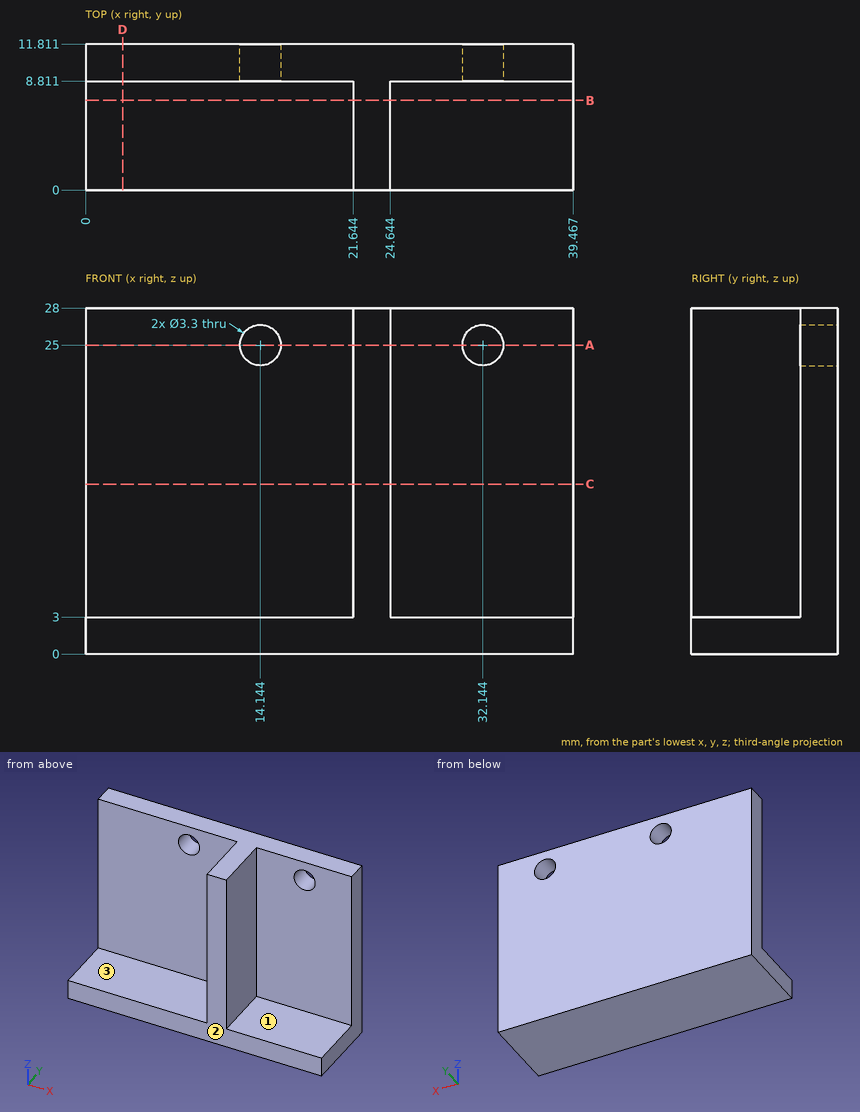
Study the drawing (mm; zero at the part's minimum x, y, z) and answer. A direction names the side the tool comes from. Coordinates: 2 decimals unless noted, no trailing zeros. Write each loop counter-clockwise with the first axis right and the second up, starting at its lowest first coordinate (ties: lowest second). Pieces come first, ordered by that corner, then holes. Notation, with made-up numbers: (-35.5, 67) - (-9.5, 67) arc R16 ccw to (-9.5, 82) - close; hole circle Ø6 at (59, 31). An arc over 180 degrees is marked (long way). Return JSON: item names as keys, results as strings. Group by question number.
1. Given pin 1 (4.5 mm diameter, centred on y = 5, z = 17, fed in from +X); pin 2 (2.5 mm diameter, centred on y = 2.5, z = 20.5, fed in from -X); pin 3 (5.5 mm diameter, centred on x = 32.14, z = 25, fed in from -Y); pin 4 (4.5 mm diameter, centred on x = 14.14, z = 25, fed in from +Y), each flat-ended and moving along its own axis, determine where each tip first touches the part or whether it passes through.
2. A cutting plane is placed at A-A, the plane z = 25. Determine the outline of the cut face in (x, y) (1 decimal).
3. A cutting plane is placed at C-C, the plane z = 13.75. Determine the outline of the cut face in (x, y) (1 decimal), plus the area to 3 significant figures.
4. Which of the six approach directions +Z, -Z, +X, -X, +Y, -Y give full straight-line access (tool end or side, diameter ignored) to the marked faces 1, 2 and 3?
5. Straight lines are drawn through the part: L1, parallel to X at y = 10.75, z = 25 (1 decimal); L2, parallel to Y at x = 17.5, z = 23; L3, parallel to X at y = 4, z = 20.5 (1 decimal). For each, find the intervals that lie inside material, in ascending order.
6. A cutting plane is placed at D-D, the plane x = 3. Determine the outline of the cut face in (y, z).
7. A cutting plane is placed at B-B, the plane y = 7.25. Determine the outline of the cut face in (x, z) (1 decimal).
Ans:
{
 "1": {"pin 1": "x = 24.64", "pin 2": "x = 21.64", "pin 3": "y = 8.81", "pin 4": "y = 11.81"},
 "2": {"outline": "(0, 8.8) - (12.5, 8.8) - (12.5, 11.8) - (0, 11.8) - close; (15.8, 8.8) - (21.6, 8.8) - (21.6, 0) - (24.6, 0) - (24.6, 8.8) - (30.5, 8.8) - (30.5, 11.8) - (15.8, 11.8) - close; (33.8, 8.8) - (39.5, 8.8) - (39.5, 11.8) - (33.8, 11.8) - close"},
 "3": {"outline": "(0, 8.8) - (21.6, 8.8) - (21.6, 0) - (24.6, 0) - (24.6, 8.8) - (39.5, 8.8) - (39.5, 11.8) - (0, 11.8) - close", "area": "145 mm²"},
 "4": {"face 1": "+Z, +X, -Y", "face 2": "+Z, -Z, +X, -X, -Y", "face 3": "+Z, -X, -Y"},
 "5": {"L1": "0 to 12.5, 15.8 to 30.5, 33.8 to 39.5", "L2": "8.81 to 11.81", "L3": "21.6 to 24.6"},
 "6": {"outline": "(0, 0) - (11.81, 0) - (11.81, 28) - (8.81, 28) - (8.81, 3) - (0, 3) - close"},
 "7": {"outline": "(0, 0) - (39.5, 0) - (39.5, 3) - (24.6, 3) - (24.6, 28) - (21.6, 28) - (21.6, 3) - (0, 3) - close"}
}
